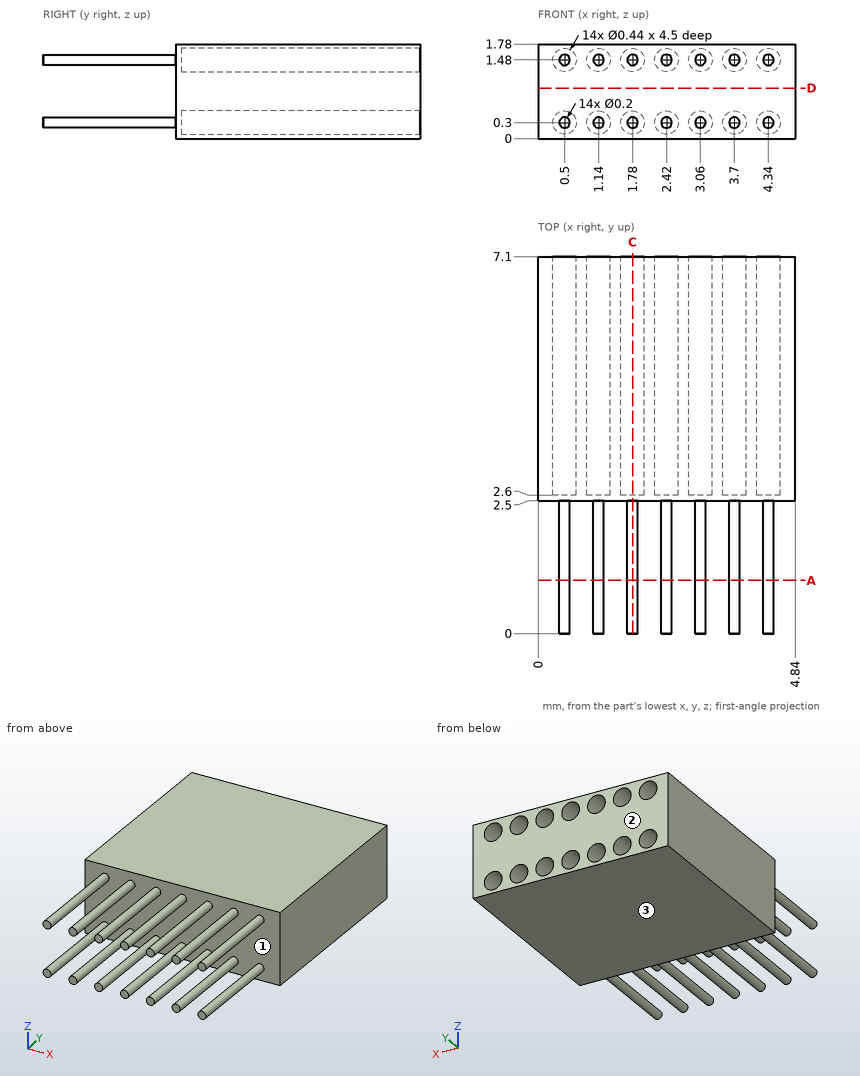
Answer from the drawing. Dimensions are ordinates in mm from the lowest x, y and z of the part. Round coordinates to 2 decimals unless told otherwise and drop trailing zeros. Write each loop counter-clockwise with the first axis right and the second up, starting at its lowest first coordinate (ties: lowest second). Pieces come first, ordered by that corner, then holes. Notation, with made-up numbers: (-3, 83.25) -> (30, 83.25) arc R36 ccw to (30, 120.25) -> close; hole circle Ø9 at (-24, -9.5). An arc over 180 degrees is marked (long way). Answer in a Markdown table with one row per item. Add a question column.
1) Find section C-C, the plane x = 1.78. Determine the outline of the cut face in (y, z), and give its area (3 significant figures).
2) Consider line 1 (Y direction, x = 0.95, z = 1). Determine where the line is inside the solid, lowest interval first.
3) Determine the mould class of the marked faces 1, 2 and 3 for opening direction Z: pulls with the +Z half, pulls with the -Z half, needs draft (parallel to the pull), parting line crosses it, or undercut.
4) Find section A-A, the plane y = 1. State how many separate pieces and enclosed holes the cut face has, and give its area (3 significant figures).
5) Given P1, Ø0.5, axis at x = 4.5, z = 1.5, coming from the +Y side, flat-ended and moving along its own axis, determine where the tip first touches the part or whether it passes through.
6) Find section D-D, the plane z = 0.95. Determine the outline of the cut face in (x, y).
Findings below:
| question | item | result |
|---|---|---|
| 1 | outline | (0, 0.2) -> (2.5, 0.2) -> (2.5, 0) -> (7.1, 0) -> (7.1, 0.08) -> (2.6, 0.08) -> (2.6, 0.52) -> (7.1, 0.52) -> (7.1, 1.26) -> (2.6, 1.26) -> (2.6, 1.7) -> (7.1, 1.7) -> (7.1, 1.78) -> (2.5, 1.78) -> (2.5, 1.58) -> (0, 1.58) -> (0, 1.38) -> (2.5, 1.38) -> (2.5, 0.4) -> (0, 0.4) -> close |
| 1 | area | 5.23 mm² |
| 2 | line 1 | 2.5 to 7.1 |
| 3 | face 1 | undercut |
| 3 | face 2 | needs draft |
| 3 | face 3 | pulls with the -Z half |
| 4 | separate pieces | 14 |
| 4 | enclosed holes | 0 |
| 4 | area | 0.440 mm² |
| 5 | P1 | y = 7.1 |
| 6 | outline | (0, 2.5) -> (4.84, 2.5) -> (4.84, 7.1) -> (0, 7.1) -> close |
